Check sheet for the modelled part. Datum: model origin and axes. Units: mm. A direction names the side the tool comes from. Round coordinates to 2 decimals unless told otherwise and drop trailing zeros. Write each loop counter-clockwise with the first axis right and the second up, starting at its lowest first coordinate (ties: lowest second). Pieces come first, ordered by that corner, then holes.
Item 1: Section check C-C, the plane z = 1.4. Record the cut outline in (x, y), plus the area to 3 significant figures.
Item 2: Depth check by flat-ended pin: pin 1 (0.6 mm diameter, centred on y = -39, z = 1, fed in from +X); pin 2 (0.6 mm diameter, centred on x = 16.5, z = 1, fed in from -Y); pin 3 (12 mm diameter, centred on x = 53, y = -32, fed in from -Z). Enter the tip coordinate at first touch or a pass-through.
Item 3: Material ranges on line 1 along Y through (x, z) = (35, 1.3); line 2 along Y through (x, z) = (5, 0.9); line 3 along X through (y, z) = (-40, 0.6), recorded low to high.
Item 4: Release check for a two-part mould opening along Y. For faces 4 (the cylindrical face through (43.1, -15.57, 1.01)), 5 (the flat face through (35, -14, 2)), 6 (the cylindrical face through (0.57, -0.6, 1.01)), 7 (the cylindrical face through (7.1, -6.84, 0.99)) record: pulls with the +Y half, pulls with the -Y half, needs draft (parallel to the pull), parting line crosses it, or undercut.
Item 5: Set-up check for faces 1 (the flat face through (42.5, -33, 1)), 2 (the flat face through (14, -15, 1)), 3 (the cylindrical face through (34.523, -32.148, 0.986)): record each of +Z, -Z, +X, -X, +Y, -Y from which the full face is reachable in a straight line by a thin tool's end or side.
Item 6: Section check A-A, the plane y = -45. Record the cut outline in (x, z).
Item 7: Section check B-B, the plane y = -7.5. Record the cut outline in (x, z), plus the area to 3 significant figures.
Item 8: Section check D-D, the plane x = 5. Record the cut outline in (y, z), plus the area to 3 significant figures.
from build123d import *

# Parameters (mm, degrees)
SKETCH_1_W      = 27.5
SKETCH_1_H      = 15
SKETCH_1_R      = 2.2
SKETCH_1_W_2    = 15
SKETCH_1_H_2    = 36
EXTRUDE_1_DEPTH = 2
FILLET_1_R      = 2


with BuildPart() as part:
    # 草图1 → 凸台-拉伸1 (new body)
    # profile 1 of 4: a face of its own
    with BuildSketch(Plane.XY):
        with Locations((13.75, -7.5)):
            Rectangle(SKETCH_1_W, SKETCH_1_H)
        with Locations((5, -7.5)):
            Circle(SKETCH_1_R, mode=Mode.SUBTRACT)
    # profile 2 of 4: a face of its own
    with BuildSketch(Plane.XY):
        with Locations((56.25, -7.5)):
            Rectangle(SKETCH_1_W, SKETCH_1_H)
        with Locations((65, -7.5)):
            Circle(SKETCH_1_R, mode=Mode.SUBTRACT)
    # profile 3 of 4: a face of its own
    with BuildSketch(Plane.XY):
        with Locations((35, -7.5)):
            Rectangle(SKETCH_1_W_2, SKETCH_1_H)
        with Locations((35, -7.5)):
            Circle(SKETCH_1_R, mode=Mode.SUBTRACT)
    # profile 4 of 4: a face of its own
    with BuildSketch(Plane.XY):
        with Locations((35, -33)):
            Rectangle(SKETCH_1_W_2, SKETCH_1_H_2)
        with Locations((35, -45)):
            Circle(SKETCH_1_R, mode=Mode.SUBTRACT)
        with Locations((35, -30)):
            Circle(SKETCH_1_R, mode=Mode.SUBTRACT)
    extrude(amount=EXTRUDE_1_DEPTH)

    # 圆角1
    fillet_1_edges = [part.edges().sort_by_distance(p)[0] for p in [
        (0, -15, 1),
        (0, 0, 1),
        (70, 0, 1),
        (70, -15, 1),
        (42.5, -15, 1),
        (42.5, -51, 1),
        (27.5, -51, 1),
        (27.5, -15, 1),
    ]]
    fillet(fillet_1_edges, radius=FILLET_1_R)


solid = part.part
Values found:
1. outline: (0, -13) arc R2 ccw to (2, -15) - (25.5, -15) arc R2 cw to (27.5, -17) - (27.5, -49) arc R2 ccw to (29.5, -51) - (40.5, -51) arc R2 ccw to (42.5, -49) - (42.5, -17) arc R2 cw to (44.5, -15) - (68, -15) arc R2 ccw to (70, -13) - (70, -2) arc R2 ccw to (68, 0) - (2, 0) arc R2 ccw to (0, -2) - close; hole circle Ø4.4 at (5, -7.5); hole circle Ø4.4 at (35, -45); hole circle Ø4.4 at (35, -30); hole circle Ø4.4 at (35, -7.5); hole circle Ø4.4 at (65, -7.5)
1. area: 1,510 mm2
2. pin 1: stops at x = 42.5
2. pin 2: stops at y = -15
2. pin 3: passes through
3. line 1: y = -51 to -47.2, -42.8 to -32.2, -27.8 to -9.7, -5.3 to 0
3. line 2: y = -15 to -9.7, -5.3 to 0
3. line 3: x = 27.5 to 42.5
4. face 4: pulls with the -Y half
4. face 5: needs draft
4. face 6: pulls with the +Y half
4. face 7: undercut
5. face 1: +Z, -Z, +X, -Y
5. face 2: +Z, -Z, -X, -Y
5. face 3: +Z, -Z
6. outline: (27.5, 0) - (32.8, 0) - (32.8, 2) - (27.5, 2) - close; (37.2, 0) - (42.5, 0) - (42.5, 2) - (37.2, 2) - close
7. outline: (0, 0) - (2.8, 0) - (2.8, 2) - (0, 2) - close; (7.2, 0) - (32.8, 0) - (32.8, 2) - (7.2, 2) - close; (37.2, 0) - (62.8, 0) - (62.8, 2) - (37.2, 2) - close; (67.2, 0) - (70, 0) - (70, 2) - (67.2, 2) - close
7. area: 114 mm2
8. outline: (-15, 0) - (-9.7, 0) - (-9.7, 2) - (-15, 2) - close; (-5.3, 0) - (0, 0) - (0, 2) - (-5.3, 2) - close
8. area: 21.2 mm2
